Geometry check sheet. Reference: the model listing, model coordinates, mm. Face numbers are marked on the shaded views. A direction names the side the tool comes from. Give positions to 0.01 mm unless a question says otherwise; leave off trailing zeros. Write each loop counter-clockwise with the first axis right and the second up, starting at its lowest first coordinate (ties: lowest second). Pieces come first, ordered by that corner, then holes.
(1) Cross-section at B-B (x = 245). Record the boundary of the cut face in (y, z), and give its area (3 significant figures).
(2) Cross-section at A-A (z = 99.5). Record the boundary of the cut face in (x, y).
(3) Cross-section at C-C (z = 30.5). Record the boundary of the cut face in (x, y), and give its area (3 significant figures).
(4) Depth check by flat-ended pin: P1, Ø10, axis at x = 162, y = -10.5, coming from the +Z side; P2, Ø3, axis at x = 303, z = 194, coming from the -Y side; P3, Ø5, axis at x = 159, y = 4, coming from the +Z side. Enter the tip coordinate at first touch or a pass-through.
(5) Mould release check, pull along X, two halves, no side actions. Record for the marked faces 3, 4 and 5: +X half, -X half, draft (parallel to the pull), parting line (faces both ways), or undercut.
(6) Tool access check on the marked faces 1 and 2. Record the directions out of +Z, -Z, +X, -X, +Y, -Y that give a thin tool (end or side, any length) a straight path to the whole face; none if there is none.
(7) Cross-section at D-D (y = -17.5). Record the boundary of the cut face in (x, z).
(8) Thickness scan on line 1 along X through (y, z) = (5.5, 123); line 2 along X through (y, z) = (-33, 288); line 3 along Y through (x, z) = (45.5, 67.5). Record the ranges inside material, lowest first.
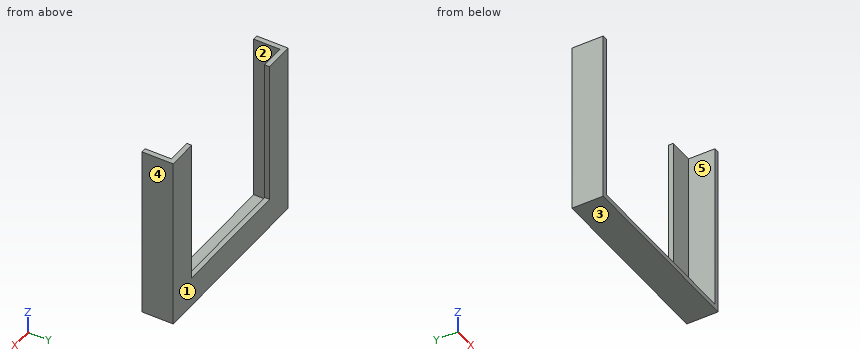
```python
from build123d import *

# Parameters (mm, degrees)
F0_W     = 353
F0_H     = 10
F1_DEPTH = 53
F2_W     = 10
F2_H     = 350
F3_DEPTH = 63
F5_DEPTH = 10


with BuildPart() as f1:
    # F0 (on Front) → F1 (new body)
    with BuildSketch(Plane.XZ):
        with Locations((176.5, 5)):
            Rectangle(F0_W, F0_H)
    extrude(amount=F1_DEPTH)

    # F2 (on face) → F3 (join)
    with BuildSketch(Plane.XZ.offset(53)):
        with Locations((358, 175)):
            Rectangle(F2_W, F2_H)
        with Locations((-5, 175)):
            Rectangle(F2_W, F2_H)
    extrude(amount=-F3_DEPTH)

    # F4 (on face) → F5 (join)
    with BuildSketch(Plane(origin=(0, 0, 0), x_dir=(-1, 0, 0), z_dir=(0, 1, 0))):
        Polygon((-353, 0), (0, 0), (0, 350), (-50, 350), (-50, 60), (-303, 60), (-303, 350), (-353, 350), align=None)
    extrude(amount=F5_DEPTH)


solid = f1.part
```
Reply:
1. outline: (-53, 0) - (10, 0) - (10, 60) - (0, 60) - (0, 10) - (-53, 10) - close
1. area: 1,130 mm2
2. outline: (-10, -53) - (0, -53) - (0, 0) - (50, 0) - (50, 10) - (-10, 10) - close; (303, 0) - (353, 0) - (353, -53) - (363, -53) - (363, 10) - (303, 10) - close
3. outline: (-10, -53) - (0, -53) - (0, 0) - (353, 0) - (353, -53) - (363, -53) - (363, 10) - (-10, 10) - close
3. area: 4,790 mm2
4. P1: stops at z = 10
4. P2: stops at y = 0
4. P3: stops at z = 60
5. face 3: draft
5. face 4: +X half
5. face 5: undercut
6. face 1: +Z, -Z, +X, -X, +Y
6. face 2: +Z, -Y
7. outline: (-10, 0) - (363, 0) - (363, 350) - (353, 350) - (353, 10) - (0, 10) - (0, 350) - (-10, 350) - close
8. line 1: x = -10 to 50, 303 to 363
8. line 2: x = -10 to 0, 353 to 363
8. line 3: y = 0 to 10
